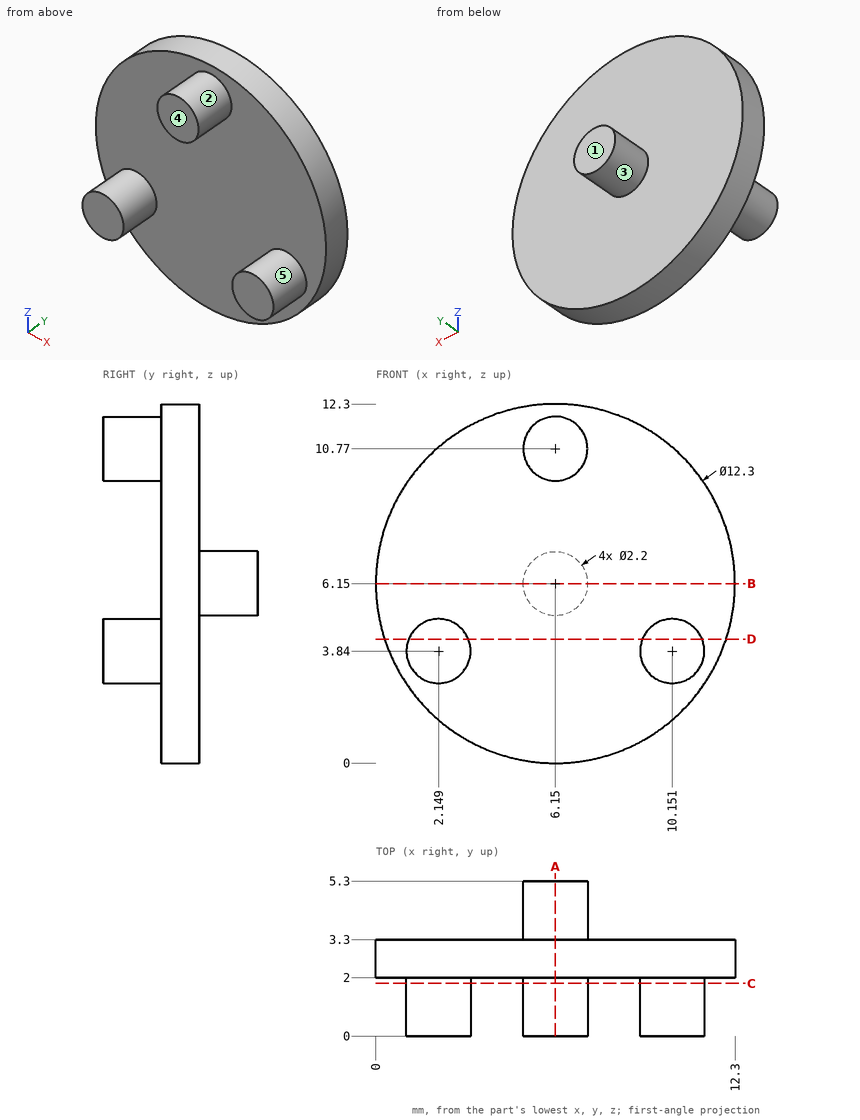
Input: dimensioned drawing with shaded views. Units: mm. Origin: part minimum x, y, z. A direction names the side the tool comes from. Give positions to 0.01 mm unless a question says otherwise; leave off trailing zeros. Write each loop counter-clockwise with the first axis right and the second up, starting at its lowest first coordinate (ties: lowest second). Pieces come first, ordered by that corner, then holes. Notation, with made-up numbers: (61.25, 81.25) - (76.25, 81.25) arc R23 cw to (76.25, 90.25) - close; hole circle Ø1 at (84, 80.5). An arc over 180 degrees is marked (long way). Write item = value, one per line. Start each with the question number.
1) Material intervals for L1, parallel to X at y = 1.85, z = 10.75; L2, parallel to Y at x = 6.5, z = 9; L3, parallel to X at y = 0.3, z = 11.25, sorted ascending. Write a range as [from, to].
2) Pin query (flat end, axial travel): pin 1 (2 mm diameter, centred on x = 3.5, z = 7, fed in from +Y); pin 2 (2 mm diameter, centred on y = 4.5, z = 10, fed in from +X). Return the tip coordinate at first contact, or that it passes through.
3) Cut plane A-A (x = 6.15). Return loops of the section in (y, z), and give its area (3 significant figures).
4) Cut plane B-B (z = 6.15). Return loops of the section in (x, y).
5) Reachability of the marked faces 1 and 2 from +Z, -Z, +X, -X, +Y, -Y: full face, straight path, thin tool, end or side. Return the list, or none.
6) Draft query along X for the marked faces 3, 4 and 5. Return one class per face: pulls with the +X half, pulls with the -X half, needs draft (parallel to the pull), parting line crosses it, or undercut.
7) Cut plane C-C (y = 1.8). Return loops of the section in (x, z), and give its area (3 significant figures).
8) Cut plane D-D (z = 4.25). Return loops of the section in (x, y).
Answers follow:
q1.L1 = [5.05, 7.25]
q1.L2 = [2, 3.3]
q1.L3 = [5.16, 7.14]
q2.pin_1 = 3.3
q2.pin_2 = through
q3.outline = (0, 9.67) - (2, 9.67) - (2, 0) - (3.3, 0) - (3.3, 5.05) - (5.3, 5.05) - (5.3, 7.25) - (3.3, 7.25) - (3.3, 12.3) - (2, 12.3) - (2, 11.87) - (0, 11.87) - close
q3.area = 24.8 mm^2
q4.outline = (0, 2) - (12.3, 2) - (12.3, 3.3) - (7.25, 3.3) - (7.25, 5.3) - (5.05, 5.3) - (5.05, 3.3) - (0, 3.3) - close
q5.face_1 = +Z, -Z, +X, -X, +Y
q5.face_2 = -Y
q6.face_3 = parting line crosses it
q6.face_4 = needs draft
q6.face_5 = undercut
q7.outline = circle Ø2.2 at (2.15, 3.84); circle Ø2.2 at (6.15, 10.77); circle Ø2.2 at (10.15, 3.84)
q7.area = 11.4 mm^2
q8.outline = (0.3, 2) - (1.13, 2) - (1.13, 0) - (3.17, 0) - (3.17, 2) - (9.13, 2) - (9.13, 0) - (11.17, 0) - (11.17, 2) - (12, 2) - (12, 3.3) - (0.3, 3.3) - close
